Part model, mm, in its own coordinate system. A direction names the side the tool comes from. Coordinates: 2 decimals unless noted, no trailing zeros. Write each loop counter-clockwise with the first axis right and the second up, starting at its lowest first coordinate (ties: lowest second). Pieces come first, ordered by that corner, then holes. Notation, with made-up numbers: M -32.5,65 L 26.5,65 A16 cw 26.5,87 Z; hole C 80,-24 d6. An arc over 180 degrees is marked long. Use a Markdown table: item, result. Add a question column.
Q1. Slice it at D-D on z = 5. Count the separate pieces of the cut face and the enclosed holes in it, then the cut area to 3 significant figures.
Q2. Pin check, flat tips, straight feed: pin 1 Ø7 at (x, y) = (18, -24.5) entering from +Z; pin 2 Ø0.6 at (y, z) = (-38, 11.5) entering from +X; pin 3 Ø5 at (x, y) = (-5, -31) entering from +Z. Stop position of each tip, or through.
Q3. Mould opens along Y. For faces 6 (the cylindrical face through (54.6, -5.42, 6.08)), 7 (the cylindrical face through (4.1, -4.216, 6.084)), 8 (the flat face through (67, -21, 6)), 9 (the cylindrical face through (-1.22, -36.716, 2.958)) say: released by +Y, released by -Y, zero draft, split by the parting line, or undercut.
Q4. Tool access for faces 1 (the flat face through (19.465, -14.535, 10.247)), 2 (the flat face through (27.369, -20.706, 8.226)), 3 (the cylindrical face through (-9, -34, 3)), 4 (the cylindrical face through (5.284, 1.22, 2.958)), 5 (the flat face through (51, -5, 11)): list every direction of +Z, -Z, +X, -X, +Y, -Y with a clear straight run to the whole face (end or side of a thin tool).
Q5. Wall check: L1, parallel to Y at x = 56.5, z = 9; L2, parallel to Y at x = 55, z = 2.5; L3, parallel to X at y = -29.5, z = 5.5. Give the ranges that are in metal, low to high. Write a range as from..to.
Q6. Slice it at B-B on y = -30. Write the cut outline in (x, z), then the cut area to 3 significant figures.
Q7. Slice it at A-A on y = -24.5. Write the cut outline in (x, z), then the cut area to 3 significant figures.
Q8. Slice it at C-C on y = 1. Write the cut outline in (x, z), then the cut area to 3 significant figures.
from build123d import *

# Parameters (mm, degrees)
F1_DEPTH    = 42
F4_DEPTH    = 2
F5_R        = 1.9
F6_DEPTH    = 12
F7_R        = 6
F8_W        = 30
F8_H        = 6
F9_DEPTH    = 10
F10_W       = 30
F10_H       = 6
F11_DEPTH   = 10
F12_W       = 50
F12_H       = 6
F13_DEPTH   = 10
F14_R       = 5
F15_R       = 2
F16_DEPTH   = 6
F17_W       = 5
F17_H       = 6
F18_DEPTH   = 0.5
F19_SIZE2   = 0.49999
F19_SIZE    = 4.99999
F19_2_SIZE2 = 0.49999
F19_2_SIZE  = 4.99999
F20_W       = 30
F20_H       = 10
F21_DEPTH   = 6
F22_R       = 4.99999


# Not quite as in the source:
# - a fillet or chamfer is up to 0.001 mm smaller than in the source, because OpenCascade refuses the exact size


with BuildPart() as f1:
    # F0 (on Front) → F1 (new body)
    with BuildSketch(Plane.XZ):
        Polygon((0, 10), (0, 0), (62, 0), (62, 10), (36, 10), (33.3, 6.5), (28.7, 6.5), (26, 10), align=None)
    extrude(amount=F1_DEPTH)

    # F3 (on face) → F4 (join)
    with BuildSketch(Plane.XY.offset(10)):
        Polygon((0, -42), (24, -42), (24, -31), (3.5, -31), (3.5, -11), (11, -11), (11, 0), (0, 0), align=None)
        Polygon((38, -42), (62, -42), (62, 0), (51, 0), (51, -11), (58.5, -11), (58.5, -31), (38, -31), align=None)
    extrude(amount=F4_DEPTH)

    # F5 (on face) → F6 (cut, through all)
    with BuildSketch(Plane.XY.offset(12)):
        with Locations((5.5, -5.5)):
            Circle(F5_R)
        with Locations((56.5, -5.5)):
            Circle(F5_R)
        with Locations((5.5, -36.5)):
            Circle(F5_R)
        with Locations((56.5, -36.5)):
            Circle(F5_R)
    extrude(amount=-F6_DEPTH, mode=Mode.SUBTRACT)

    # F7
    f7_edges = [f1.edges().sort_by_distance(p)[0] for p in [
        (0, -42, 6),
        (0, 0, 6),
        (62, -42, 6),
        (62, 0, 6),
    ]]
    fillet(f7_edges, radius=F7_R)

    # F8 (on face) → F9 (join)
    with BuildSketch(Plane.YZ.offset(62)):
        with Locations((-21, 3)):
            Rectangle(F8_W, F8_H)
    extrude(amount=F9_DEPTH)

    # F10 (on face) → F11 (join)
    with BuildSketch(Plane(origin=(0, 0, 0), x_dir=(0, -1, 0), z_dir=(-1, 0, 0))):
        with Locations((21, 3)):
            Rectangle(F10_W, F10_H)
    extrude(amount=F11_DEPTH)

    # F12 (on face) → F13 (join)
    with BuildSketch(Plane(origin=(0, 0, 0), x_dir=(-1, 0, 0), z_dir=(0, 1, 0))):
        with Locations((-31, 3)):
            Rectangle(F12_W, F12_H)
    extrude(amount=F13_DEPTH)

    # F14
    f14_edges = [f1.edges().sort_by_distance(p)[0] for p in [
        (6, 10, 3),
        (-10, -6, 3),
        (-10, -36, 3),
        (56, 10, 3),
        (72, -6, 3),
        (72, -36, 3),
        (6, 0, 9),
        (6, 0, 3),
        (0, -6, 9),
        (0, -6, 3),
        (0, -36, 9),
        (0, -36, 3),
        (56, 0, 9),
        (56, 0, 3),
        (62, -6, 9),
        (62, -6, 3),
        (62, -36, 3),
        (62, -36, 9),
    ]]
    fillet(f14_edges, radius=F14_R)

    # F15 (on face) → F16 (cut, through all)
    with BuildSketch(Plane.XY.offset(6)):
        with Locations((-5, -11)):
            Circle(F15_R)
        with Locations((-5, -31)):
            Circle(F15_R)
        with Locations((11, 5)):
            Circle(F15_R)
        with Locations((51, 5)):
            Circle(F15_R)
        with Locations((67, -11)):
            Circle(F15_R)
        with Locations((67, -31)):
            Circle(F15_R)
    extrude(amount=-F16_DEPTH, mode=Mode.SUBTRACT)

    # F17 (on face) → F18 (join)
    with BuildSketch(Plane.XY.offset(10)):
        with Locations((19.5, -14)):
            Rectangle(F17_W, F17_H)
        with Locations((42.5, -14)):
            Rectangle(F17_W, F17_H)
    extrude(amount=F18_DEPTH)

    # F19 (size 5 and 0.5 in the source; OpenCascade refuses exactly that, so slightly less here)
    f19_edges = [f1.edges().sort_by_distance(p)[0] for p in [
        (19.5, -17, 10.5),
    ]]
    f19_side = f1.faces().sort_by_distance((19.5, -14, 10.5))[0]
    chamfer(f19_edges, length=F19_SIZE, length2=F19_SIZE2, reference=f19_side)

    # F19#2 (size 5 and 0.5 in the source; OpenCascade refuses exactly that, so slightly less here)
    f19_2_edges = [f1.edges().sort_by_distance(p)[0] for p in [
        (42.5, -17, 10.5),
    ]]
    f19_2_side = f1.faces().sort_by_distance((42.5, -14, 10.5))[0]
    chamfer(f19_2_edges, length=F19_2_SIZE, length2=F19_2_SIZE2, reference=f19_2_side)

    # F20 (on face) → F21 (cut, through all)
    with BuildSketch(Plane.XY.offset(6)):
        with Locations((31, 5)):
            Rectangle(F20_W, F20_H)
    extrude(amount=-F21_DEPTH, mode=Mode.SUBTRACT)

    # F22 (radius 5 in the source; OpenCascade refuses exactly that, so slightly less here)
    f22_edges = [f1.edges().sort_by_distance(p)[0] for p in [
        (16, 10, 3),
        (46, 10, 3),
        (16, 0, 3),
        (46, 0, 3),
    ]]
    fillet(f22_edges, radius=F22_R)


solid = f1.part
Recorded:
| question | item | result |
|---|---|---|
| 1 | separate pieces | 1 |
| 1 | enclosed holes | 10 |
| 1 | area | 3,230 mm² |
| 2 | pin 1 | z = 10 |
| 2 | pin 2 | x = 61.75 |
| 2 | pin 3 | z = 6 |
| 3 | face 6 | undercut |
| 3 | face 7 | undercut |
| 3 | face 8 | zero draft |
| 3 | face 9 | released by -Y |
| 4 | face 1 | +Z |
| 4 | face 2 | +Z, +Y, -Y |
| 4 | face 3 | +Z, -Z, -X, -Y |
| 4 | face 4 | +Z, -Z, -X, +Y |
| 4 | face 5 | +Z, +Y |
| 5 | L1 | -41.98..-38.4, -34.6..-7.4, -3.6..-0.02 |
| 5 | L2 | -42..-37.67, -35.33..-6.67, -4.33..8 |
| 5 | L3 | -10..-6.32, -3.68..65.68, 68.32..72 |
| 6 | outline | M -10,0 L -6.73,0 L -6.73,6 L -10,6 Z; M -3.27,0 L 65.27,0 L 65.27,6 L 62,6 L 62,12 L 58.5,12 L 58.5,10 L 36,10 L 33.3,6.5 L 28.7,6.5 L 26,10 L 3.5,10 L 3.5,12 L 0,12 L 0,6 L -3.27,6 Z; M 68.73,0 L 72,0 L 72,6 L 68.73,6 Z |
| 6 | area | 687 mm² |
| 7 | outline | M -10,0 L 72,0 L 72,6 L 62,6 L 62,12 L 58.5,12 L 58.5,10 L 36,10 L 33.3,6.5 L 28.7,6.5 L 26,10 L 3.5,10 L 3.5,12 L 0,12 L 0,6 L -10,6 Z |
| 7 | area | 728 mm² |
| 8 | outline | M 5.14,0 L 18,0 L 18,6 L 5.14,6 Z; M 44,0 L 56.86,0 L 56.86,6 L 44,6 Z |
| 8 | area | 154 mm² |
